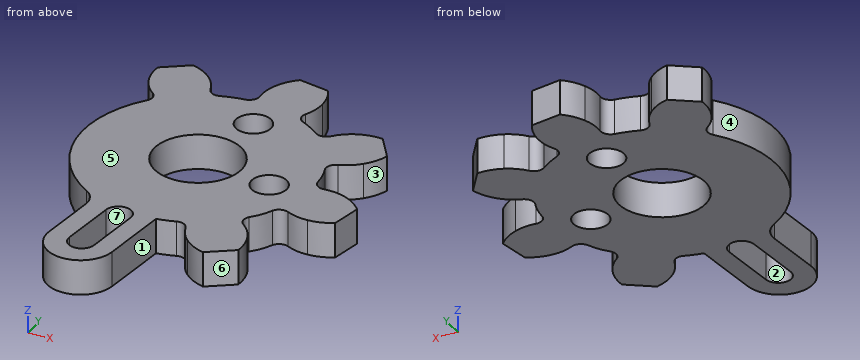
```python
from build123d import *

# Parameters (mm, degrees)
ESQUISSE1_R               = 3.7
ESQUISSE1_R_2             = 1.5
T_LE_DE_BASE_PLI_E1_DEPTH = 3


# Sheet-metal steps are written as plain solids
with BuildPart() as part:
    # Esquisse1 → Tôle de base pliée1 (new body)
    with BuildSketch(Plane.XY):
        with BuildLine():
            Line((1343.247008076, 1938.302325501), (1345.89746161, 1937.787450694))
            ThreePointArc((1345.89746161, 1937.787450694), (1346.302249899, 1936.788677026), (1346.449670341, 1935.72112393))
            ThreePointArc((1346.449670341, 1935.72112393), (1346.342555269, 1934.751830987), (1346.001938932, 1933.838056967))
            ThreePointArc((1346.001938932, 1933.838056967), (1345.945060229, 1933.190654063), (1346.362467863, 1932.692520976))
            ThreePointArc((1346.362467863, 1932.692520976), (1347.233633787, 1932.178943437), (1348.046916436, 1931.57789162))
            ThreePointArc((1348.046916436, 1931.57789162), (1348.668588775, 1931.388447146), (1349.242230693, 1931.693898708))
            ThreePointArc((1349.242230693, 1931.693898708), (1349.950118086, 1932.364642987), (1350.800392256, 1932.842174436))
            ThreePointArc((1350.800392256, 1932.842174436), (1351.840616067, 1933.123842365), (1352.918151311, 1933.141736383))
            Line((1352.918151311, 1933.141736383), (1354.428233511, 1930.903511249))
            ThreePointArc((1354.428233511, 1930.903511249), (1354.008222422, 1929.911043071), (1353.357590382, 1929.051927044))
            ThreePointArc((1353.357590382, 1929.051927044), (1352.596454976, 1928.442275224), (1351.709467048, 1928.03699154))
            ThreePointArc((1351.709467048, 1928.03699154), (1351.211464748, 1927.619427873), (1351.154383232, 1926.97204282))
            ThreePointArc((1351.154383232, 1926.97204282), (1351.440459119, 1925.999644606), (1351.557306264, 1924.992795836))
            ThreePointArc((1351.557306264, 1924.992795836), (1351.862937519, 1924.419249637), (1352.48455048, 1924.229610418))
            ThreePointArc((1352.48455048, 1924.229610418), (1353.459390284, 1924.203346271), (1354.398290641, 1923.939777365))
            ThreePointArc((1354.398290641, 1923.939777365), (1355.333009255, 1923.403397357), (1356.107594714, 1922.65411786))
            Line((1356.107594714, 1922.65411786), (1355.592719908, 1920.003664327))
            ThreePointArc((1355.592719908, 1920.003664327), (1354.59394624, 1919.598876037), (1353.526393144, 1919.451455596))
            ThreePointArc((1353.526393144, 1919.451455596), (1352.557100201, 1919.558570667), (1351.643326181, 1919.899187005))
            ThreePointArc((1351.643326181, 1919.899187005), (1350.995923277, 1919.956065707), (1350.497790189, 1919.538658073))
            ThreePointArc((1350.497790189, 1919.538658073), (1350.024286618, 1918.640974498), (1349.383160833, 1917.854209501))
            ThreePointArc((1349.383160833, 1917.854209501), (1349.19371636, 1917.232537161), (1349.499167922, 1916.658895244))
            ThreePointArc((1349.499167922, 1916.658895244), (1350.169912201, 1915.951007851), (1350.64744365, 1915.100733681))
            ThreePointArc((1350.64744365, 1915.100733681), (1350.929111579, 1914.06050987), (1350.947005597, 1912.982974625))
            Line((1350.947005597, 1912.982974625), (1348.708780463, 1911.472892426))
            ThreePointArc((1348.708780463, 1911.472892426), (1347.716312285, 1911.892903515), (1346.857196258, 1912.543535554))
            ThreePointArc((1346.857196258, 1912.543535554), (1346.247544438, 1913.304670961), (1345.842260754, 1914.191658889))
            ThreePointArc((1345.842260754, 1914.191658889), (1345.424697087, 1914.689661189), (1344.777312034, 1914.746742704))
            ThreePointArc((1344.777312034, 1914.746742704), (1344.006653047, 1914.538715485), (1343.221559749, 1914.394427185))
            Line((1343.221559749, 1914.394427185), (1342.565641761, 1908.368090699))
            ThreePointArc((1342.565641761, 1908.368090699), (1339.42399637, 1905.843201744), (1336.899107414, 1908.984847135))
            Line((1336.899107414, 1908.984847135), (1337.442443377, 1913.976820816))
            ThreePointArc((1337.442443377, 1913.976820816), (1337.260922483, 1915.05095745), (1336.54337922, 1915.870622631))
            ThreePointArc((1336.54337922, 1915.870622631), (1332.217504298, 1922.559333364), (1334.323234317, 1930.241647222))
            ThreePointArc((1334.323234317, 1930.241647222), (1334.51267879, 1930.863319562), (1334.207227229, 1931.436961479))
            ThreePointArc((1334.207227229, 1931.436961479), (1333.536482949, 1932.144848872), (1333.0589515, 1932.995123042))
            ThreePointArc((1333.0589515, 1932.995123042), (1332.777283571, 1934.035346853), (1332.759389553, 1935.112882097))
            Line((1332.759389553, 1935.112882097), (1334.997614687, 1936.622964297))
            ThreePointArc((1334.997614687, 1936.622964297), (1335.990082865, 1936.202953208), (1336.849198892, 1935.552321168))
            ThreePointArc((1336.849198892, 1935.552321168), (1337.458850712, 1934.791185762), (1337.864134396, 1933.904197834))
            ThreePointArc((1337.864134396, 1933.904197834), (1338.281698063, 1933.406195534), (1338.929083116, 1933.349114018))
            ThreePointArc((1338.929083116, 1933.349114018), (1339.908244608, 1933.601967191), (1340.9083301, 1933.752037051))
            ThreePointArc((1340.9083301, 1933.752037051), (1341.481876299, 1934.057668306), (1341.671515518, 1934.679281266))
            ThreePointArc((1341.671515518, 1934.679281266), (1341.697779666, 1935.65412107), (1341.961348571, 1936.593021428))
            ThreePointArc((1341.961348571, 1936.593021428), (1342.497728579, 1937.527740041), (1343.247008076, 1938.302325501))
        make_face()
        with Locations((1341.853197575, 1924.047928361)):
            Circle(ESQUISSE1_R, mode=Mode.SUBTRACT)
        with Locations((1343.153024926, 1930.717446866)):
            Circle(ESQUISSE1_R_2, mode=Mode.SUBTRACT)
        with Locations((1348.476026591, 1922.946328291)):
            Circle(ESQUISSE1_R_2, mode=Mode.SUBTRACT)
        with BuildLine():
            Line((1340.880246952, 1908.666985015), (1341.425079269, 1913.672706653))
            ThreePointArc((1341.425079269, 1913.672706653), (1340.438549544, 1914.900216702), (1339.211039495, 1913.913686977))
            Line((1339.211039495, 1913.913686977), (1338.666207179, 1908.907965339))
            ThreePointArc((1338.666207179, 1908.907965339), (1339.652736904, 1907.68045529), (1340.880246952, 1908.666985015))
        make_face(mode=Mode.SUBTRACT)
    extrude(amount=-T_LE_DE_BASE_PLI_E1_DEPTH)


solid = part.part
```
Verification items for the finished model (mm, model axes). Face numbers are marked on the shaded views. A direction names the side the tool comes from. Round coordinates to 2 decimals unless told otherwise and drop trailing zeros. Write each loop counter-clockwise with the first axis right and the second up, starting at its lowest first coordinate (ties: lowest second). Pieces come first, ordered by that corner, then holes.
1. Section check C-C on z = -1.45. State how many separate pieces and enclosed holes the cut face has, plus the area to 3 significant figures.
2. Section check A-A on x = 1339.75. Enter the section's corners in (y, z), plus the area to 3 significant figures.
3. Gauge pin test, flat end, axial feed: P1, Ø4, axis at x = 1348.48, y = 1922.95, coming from the +Z side. Record the tip position at first contact, or that the pin passes through.
4. Access from +Z, -Z, +X, -X, +Y, -Y to the whole of each face (thin tool, end or side, straight path). Record for the marked faces 1, 2 and 3.
5. Section check B-B on y = 1917. Enter the section's corners in (x, z), plus the area to 3 significant figures.
6. Draft check along X on the marked faces 4, 5, 6 and 7. Enter one of: +X half, -X half, draft (parallel to the pull), parting line (faces both ways), or undercut.
7. Scan lines: L1, parallel to Y at x = 1343.5, z = -0.7; L2, parallel to X at y = 1912, z = -0.5; L3, parallel to Y at x = 1340.5, z = -1.3. Record each from-to range of solid material in increasing order.
Answer:
1. separate pieces: 1
1. enclosed holes: 4
1. area: 372 mm2
2. outline: (1905.83, -3) - (1907.67, -3) - (1907.67, 0) - (1905.83, 0) - close; (1914.75, -3) - (1921, -3) - (1921, 0) - (1914.75, 0) - close; (1927.09, -3) - (1933.57, -3) - (1933.57, 0) - (1927.09, 0) - close
2. area: 43.7 mm2
3. P1: stops at z = 0
4. face 1: +Z, -Z, -Y
4. face 2: +Z, -Z
4. face 3: +Z, -Z, +X
5. outline: (1335.12, -3) - (1349.25, -3) - (1349.25, 0) - (1335.12, 0) - close
5. area: 42.4 mm2
6. face 4: -X half
6. face 5: draft
6. face 6: +X half
6. face 7: undercut
7. L1: y = 1914.44 to 1920.73, 1927.36 to 1929.26, 1932.18 to 1938.25
7. L2: x = 1337.23 to 1339, 1341.24 to 1342.96, 1347.54 to 1349.49
7. L3: y = 1905.93 to 1907.94, 1914.89 to 1920.6, 1927.49 to 1933.7
